Answer from the drawing. Dimensions are ordinates in mm from the lowest x, y and z of the part. A direction names the side the tool comes from. Give positions to 0.01 mm unless a question says otherwise; leave off trailing zeros. Write each loop counter-clockwise with the first axis right and the second up, starting at its lowest first coordinate (ties: lowest second). Pieces come first, ordered by that corner, then holes. Notation, with made-up numbers: (31.25, -23.75) -> (56.25, -23.75) arc R8 cw to (56.25, -18.75) -> close; hole circle Ø2 at (29, 14.25). An arc over 180 degrees is marked (long way). Use a Markdown table: item, result. Add a question column.
Q1. For a pull along X with two mould halves and no side action, classify the marked faces 1, 2, 3 and 4 as pulls with the +X half, pulls with the -X half, needs draft (parallel to the pull), parting line crosses it, or undercut.
Q2. For the marked faces 5, 6 and 7, determine the directions among +Z, -Z, +X, -X, +Y, -Y from which every point of the face is accessible in a straight line to the end or side of a thin tool.
Q3. Section D-D, the plane z = 12.5 is taken. Give the vertices of the cut face in (x, y) (1 decimal), plus the area to 3 significant figures.
Q4. Section C-C, the plane x = 31.5 is taken. Give the vertices of the cut face in (y, z).
Q5. Section A-A, the plane y = 5 is taken. Give the vertices of the cut face in (x, z), plus the area to 3 significant figures.
Q6. Consider line 1 (X direction, y = 5, z = 5.75); line 2 (Z direction, x = 29.5, y = 8); line 3 (Z direction, x = 30.5, y = 5.75). Determine where each line is inside the solid, lowest interval first.
Q7. Section B-B, the plane z = 19 is taken. Give the vertices of the cut face in (x, y), plus the area to 3 significant figures.
Q8. Each of these flat-tipped pins is pushed along its axis until it touches: pin 1 Ø6 at (x, z) = (22, 9.5) entering from +Y; pin 2 Ø10 at (x, z) = (12.5, 18.5) entering from -Y (1 decimal); pin 3 Ø3 at (y, z) = (3, 17.5) entering from -X; pin 4 Ø5 at (x, z) = (29.23, 19.25) entering from -Y. Where does it stop, or does it pass through?
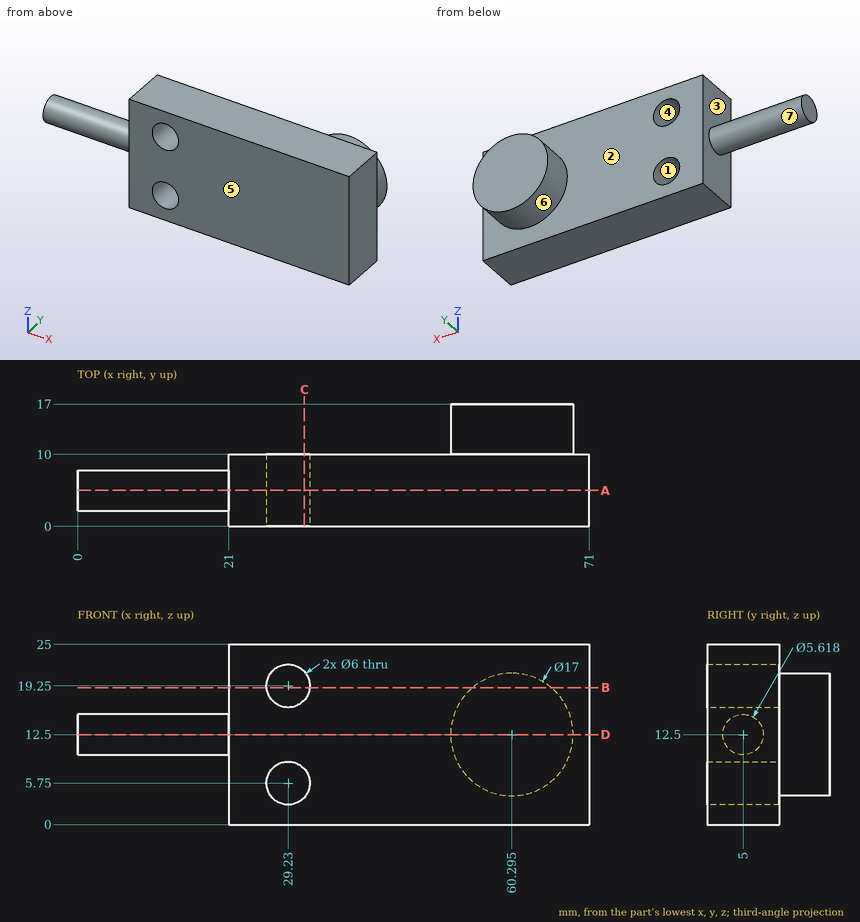
Result set:
| question | item | result |
|---|---|---|
| 1 | face 1 | undercut |
| 1 | face 2 | needs draft |
| 1 | face 3 | pulls with the -X half |
| 1 | face 4 | undercut |
| 2 | face 5 | +Z, -Z, +X, -X, -Y |
| 2 | face 6 | +Y |
| 2 | face 7 | -X |
| 3 | outline | (0, 2.2) -> (21, 2.2) -> (21, 0) -> (71, 0) -> (71, 10) -> (68.8, 10) -> (68.8, 17) -> (51.8, 17) -> (51.8, 10) -> (21, 10) -> (21, 7.8) -> (0, 7.8) -> close |
| 3 | area | 737 mm2 |
| 4 | outline | (0, 0) -> (10, 0) -> (10, 3.79) -> (0, 3.79) -> close; (0, 7.71) -> (10, 7.71) -> (10, 17.29) -> (0, 17.29) -> close; (0, 21.21) -> (10, 21.21) -> (10, 25) -> (0, 25) -> close |
| 5 | outline | (0, 9.69) -> (21, 9.69) -> (21, 0) -> (71, 0) -> (71, 25) -> (21, 25) -> (21, 15.31) -> (0, 15.31) -> close; hole circle Ø6 at (29.23, 5.75); hole circle Ø6 at (29.23, 19.25) |
| 5 | area | 1,310 mm2 |
| 6 | line 1 | x = 21 to 26.23, 32.23 to 71 |
| 6 | line 2 | z = 0 to 2.76, 8.74 to 16.26, 22.24 to 25 |
| 6 | line 3 | z = 0 to 3.03, 8.47 to 16.53, 21.97 to 25 |
| 7 | outline | (21, 0) -> (26.24, 0) -> (26.24, 10) -> (21, 10) -> close; (32.22, 0) -> (71, 0) -> (71, 10) -> (65.77, 10) -> (65.77, 17) -> (54.82, 17) -> (54.82, 10) -> (32.22, 10) -> close |
| 7 | area | 517 mm2 |
| 8 | pin 1 | stops at y = 10 |
| 8 | pin 2 | stops at y = 2.4 |
| 8 | pin 3 | stops at x = 21 |
| 8 | pin 4 | passes through |
